Check sheet for the modelled part. Datum: model origin and axes. Units: mm. Coordinates: 2 decimals unless noted, no trailing zeros. Write each loop counter-clockwise with the first axis right and the second up, starting at its lowest first coordinate (ties: lowest second). Pieces come first, ordered by that corner, then holes. Notation, with made-up numbers: (-30, 57) -> (11, 57) arc R19 cw to (11, 84) -> close; hole circle Ø2 at (80.5, 4). An arc over 180 degrees is marked (long way). One line per item, written item: value. Start each with the question number.
1) Scan lines: line 1 along X through (y, z) = (-0.1, 14.5); line 2 along Z through (x, y) = (-56, -0.25); line 3 along X through (y, z) = (-0.3, 19.25). Record each from-to range of solid material in increasing order. Write a range as [from, to].
2) Sectioned sample at A-A on z = 2.5. Enter the section's corners in (x, y), plus the area to 3 significant figures.
3) Sectioned sample at C-C on x = 10. Enter the section's corners in (y, z), plus the area to 3 significant figures.
4) Sectioned sample at B-B on y = -0.4. Enter the section's corners in (x, z), plus the area to 3 significant figures.
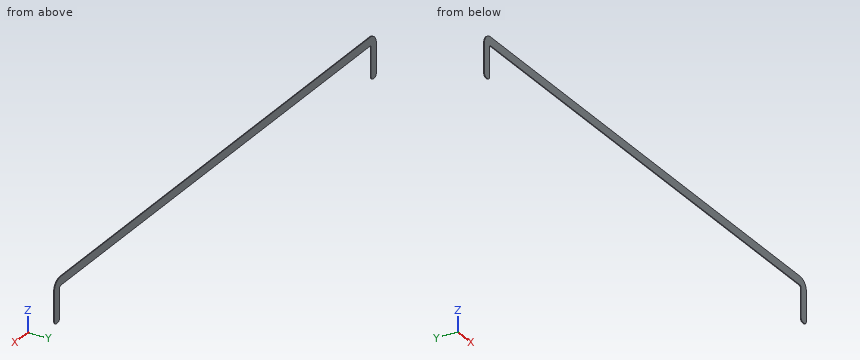
```python
from build123d import *

# Parameters (mm, degrees)
F1_DEPTH = 0.5


with BuildPart() as f1:
    # F0 (on Front) → F1 (new body)
    with BuildSketch(Plane.XZ):
        with BuildLine():
            ThreePointArc((-150.898975, -4.798244), (-149.484761, -4.212457), (-148.898975, -2.798244))
            Line((-148.898975, -2.798244), (-148.898975, 14.201756))
            ThreePointArc((-148.898975, 14.201756), (-148.606081, 14.908863), (-147.898975, 15.201756))
            Line((-147.898975, 15.201756), (150.101025, 15.201756))
            ThreePointArc((150.101025, 15.201756), (150.808132, 14.908863), (151.101025, 14.201756))
            Line((151.101025, 14.201756), (151.101025, -2.798244))
            ThreePointArc((151.101025, -2.798244), (151.686812, -4.212457), (153.101025, -4.798244))
            Line((153.101025, -4.798244), (154.101025, -4.798244))
            ThreePointArc((154.101025, -4.798244), (155.515239, -4.212457), (156.101025, -2.798244))
            Line((156.101025, -2.798244), (156.101025, 14.201756))
            ThreePointArc((156.101025, 14.201756), (154.343666, 18.444397), (150.101025, 20.201756))
            Line((150.101025, 20.201756), (-147.898975, 20.201756))
            ThreePointArc((-147.898975, 20.201756), (-152.141615, 18.444397), (-153.898975, 14.201756))
            Line((-153.898975, 14.201756), (-153.898975, -2.798244))
            ThreePointArc((-153.898975, -2.798244), (-153.313188, -4.212457), (-151.898975, -4.798244))
            Line((-151.898975, -4.798244), (-150.898975, -4.798244))
        make_face()
    extrude(amount=F1_DEPTH)


solid = f1.part
```
Answers:
1. line 1: x = [-153.89, -148.85], [151.06, 156.09]
1. line 2: z = [15.2, 20.2]
1. line 3: x = [-151.14, 153.34]
2. outline: (-153.9, -0.5) -> (-148.9, -0.5) -> (-148.9, 0) -> (-153.9, 0) -> close; (151.1, -0.5) -> (156.1, -0.5) -> (156.1, 0) -> (151.1, 0) -> close
2. area: 5.00 mm2
3. outline: (-0.5, 15.2) -> (0, 15.2) -> (0, 20.2) -> (-0.5, 20.2) -> close
3. area: 2.50 mm2
4. outline: (-153.9, -2.8) arc R2 ccw to (-151.9, -4.8) -> (-150.9, -4.8) arc R2 ccw to (-148.9, -2.8) -> (-148.9, 14.2) arc R1 cw to (-147.9, 15.2) -> (150.1, 15.2) arc R1 cw to (151.1, 14.2) -> (151.1, -2.8) arc R2 ccw to (153.1, -4.8) -> (154.1, -4.8) arc R2 ccw to (156.1, -2.8) -> (156.1, 14.2) arc R6 ccw to (150.1, 20.2) -> (-147.9, 20.2) arc R6 ccw to (-153.9, 14.2) -> close
4. area: 1,730 mm2
